from build123d import *

# Parameters (mm, degrees)
SKETCH1_W           = 20
SKETCH1_H           = 6.7
BOSS_EXTRUDE1_DEPTH = 1.5
SKETCH2_R           = 1.15
CUT_EXTRUDE1_DEPTH  = 1.5
BOSS_EXTRUDE2_DEPTH = 5
BOSS_EXTRUDE3_START = -1
BOSS_EXTRUDE3_DEPTH = 1
SKETCH5_W           = 6
SKETCH5_H           = 0.6
BOSS_EXTRUDE4_DEPTH = 4.5
SKETCH6_W           = 9
SKETCH6_H           = 1
BOSS_EXTRUDE5_DEPTH = 7.5


with BuildPart() as part:
    # Sketch1 → Boss-Extrude1 (new body)
    with BuildSketch(Plane.XY):
        Rectangle(SKETCH1_W, SKETCH1_H)
    extrude(amount=BOSS_EXTRUDE1_DEPTH)

    # Sketch2 → Cut-Extrude1 (cut)
    with BuildSketch(Plane(origin=(0, 0, 0), x_dir=(-1, 0, 0), z_dir=(0, 0, -1))):
        with Locations((-8, 0)):
            Circle(SKETCH2_R)
        with Locations((8, 0)):
            Circle(SKETCH2_R)
        with BuildLine():
            Line((-3, 1.25), (3, 1.25))
            ThreePointArc((3, 1.25), (4.25, 0), (3, -1.25))
            Line((3, -1.25), (-3, -1.25))
            ThreePointArc((-3, -1.25), (-4.25, 0), (-3, 1.25))
        make_face()
    extrude(amount=-CUT_EXTRUDE1_DEPTH, mode=Mode.SUBTRACT)

    # Sketch3 → Boss-Extrude2 (add)
    with BuildSketch(Plane.XY.offset(1.5)):
        with BuildLine():
            Line((3, 1.35), (-3, 1.35))
            ThreePointArc((-3, 1.35), (-4.35, 0), (-3, -1.35))
            Line((-3, -1.35), (3, -1.35))
            ThreePointArc((3, -1.35), (4.35, 0), (3, 1.35))
        make_face()
        with BuildLine():
            Line((3, 1.25), (-3, 1.25))
            ThreePointArc((-3, 1.25), (-4.25, 0), (-3, -1.25))
            Line((-3, -1.25), (3, -1.25))
            ThreePointArc((3, -1.25), (4.25, 0), (3, 1.25))
        make_face(mode=Mode.SUBTRACT)
    extrude(amount=BOSS_EXTRUDE2_DEPTH)

    # Sketch4 → Boss-Extrude3 (add)
    with BuildSketch(Plane.XY.offset(6.5).offset(BOSS_EXTRUDE3_START)):
        with BuildLine():
            Line((3, 1.35), (-3, 1.35))
            ThreePointArc((-3, 1.35), (-4.35, 0), (-3, -1.35))
            Line((-3, -1.35), (3, -1.35))
            ThreePointArc((3, -1.35), (4.35, 0), (3, 1.35))
        make_face()
    extrude(amount=BOSS_EXTRUDE3_DEPTH)

    # Sketch5 → Boss-Extrude4 (add)
    with BuildSketch(Plane(origin=(0, 0, 5.5), x_dir=(-1, 0, 0), z_dir=(0, 0, -1))):
        Rectangle(SKETCH5_W, SKETCH5_H)
    extrude(amount=BOSS_EXTRUDE4_DEPTH)

    # Sketch6 → Boss-Extrude5 (add)
    with BuildSketch(Plane.XY.offset(6.5)):
        Rectangle(SKETCH6_W, SKETCH6_H)
    extrude(amount=BOSS_EXTRUDE5_DEPTH)


solid = part.part
CAD build for the part. Positions are in the model's coordinates, mm. A direction names the side the tool comes from. Give positions to 0.01 mm unless a question says otherwise; leave off trailing zeros. Loops run counter-clockwise (first coordinate to the right, second up) from the corner with the lowest first, then second, coordinate; pieces in that order, holes last. Notation, with made-up numbers: M 71,-11 L 104,-11 A18 ccw 104,-4 Z; hole C 75,83 d5. An arc over 180 degrees is marked long. Answer in a Markdown table with one row per item. Add a question column.
Item 1: Drop flat-ended pins along their axis: P1, Ø0.7, axis at y = 0, z = 2, coming from the +X side; P2, Ø1, axis at x = -0.5, z = 10, coming from the +Y side; P3, Ø0.8, axis at y = 0, z = 9, coming from the +X side; P4, Ø5, axis at x = -1, z = 2.5, coming from the -Y side. Give the stop position or say it passes through.
Item 2: Band-saw the part on B-B on x = 8. Give the cut face in (y, z), then the cut area to 3 significant figures.
Item 3: Band-saw the part on A-A on z = 4.75. Give the cut face in (x, y), then the cut area to 3 significant figures.
Item 4: Mould opens along Y. For faces 6 (the face through (0, 1, 6.5)), 7 (the face through (0, -0.5, 10)), 8 (the face through (0, 0.3, 3)) say: +Y half, -Y half, draft (parallel to the pull), parting line (faces both ways), or undercut.
Item 5: Tool access for faces 1 (the face through (-4.5, 0, 10)), 2 (the face through (4.5, 0, 10)), 3 (the face through (-10, 0, 1)), 4 (the face through (0, -0.3, 3)), 5 (the face through (0, -1, 6.5)): list every direction of +Z, -Z, +X, -X, +Y, -Y with a clear straight run to the whole face (end or side of a thin tool).
Item 6: Band-saw the part on C-C on y = 0. Give the cut face in (x, z), then the cut area to 3 significant figures.
Item 7: Probe probe 1 along Y at (x, z) = (-8, 0.75); probe 2 along Y at (x, z) = (-2.5, 9); probe 3 along Z at (x, y) = (-3.25, -0.25). List the from-to ranges inside material, lowest first.
Item 8: Band-saw the part on D-D on x = 2. Give the cut face in (y, z).
Reply:
| question | item | result |
|---|---|---|
| 1 | P1 | stops at x = 4.35 |
| 1 | P2 | stops at y = 0.5 |
| 1 | P3 | stops at x = 4.5 |
| 1 | P4 | stops at y = -3.35 |
| 2 | outline | M -3.35,0 L -1.15,0 L -1.15,1.5 L -3.35,1.5 Z; M 1.15,0 L 3.35,0 L 3.35,1.5 L 1.15,1.5 Z |
| 2 | area | 6.60 mm^2 |
| 3 | outline | M -3,-1.35 L 3,-1.35 A1.35 ccw 3,1.35 L -3,1.35 A1.35 ccw Z; M -3,-0.3 L 3,-0.3 L 3,0.3 L -3,0.3 Z; hole M -3,-1.25 L 3,-1.25 A1.25 ccw 3,1.25 L -3,1.25 A1.25 ccw Z |
| 3 | area | 5.62 mm^2 |
| 4 | face 6 | draft |
| 4 | face 7 | -Y half |
| 4 | face 8 | undercut |
| 5 | face 1 | +Z, -X, +Y, -Y |
| 5 | face 2 | +Z, +X, +Y, -Y |
| 5 | face 3 | +Z, -Z, -X, +Y, -Y |
| 5 | face 4 | -Z |
| 5 | face 5 | +Z, +X, -X, -Y |
| 6 | outline | M -10,0 L -9.15,0 L -9.15,1.5 L -10,1.5 Z; M -6.85,0 L -4.25,0 L -4.25,5.5 L -3,5.5 L -3,1 L 3,1 L 3,5.5 L 4.25,5.5 L 4.25,0 L 6.85,0 L 6.85,1.5 L 4.35,1.5 L 4.35,6.5 L 4.5,6.5 L 4.5,14 L -4.5,14 L -4.5,6.5 L -4.35,6.5 L -4.35,1.5 L -6.85,1.5 Z; M 9.15,0 L 10,0 L 10,1.5 L 9.15,1.5 Z |
| 6 | area | 114 mm^2 |
| 7 | probe 1 | y = -3.35 to -1.15, 1.15 to 3.35 |
| 7 | probe 2 | y = -0.5 to 0.5 |
| 7 | probe 3 | z = 5.5 to 14 |
| 8 | outline | M -3.35,0 L -1.25,0 L -1.25,5.5 L -0.3,5.5 L -0.3,1 L 0.3,1 L 0.3,5.5 L 1.25,5.5 L 1.25,0 L 3.35,0 L 3.35,1.5 L 1.35,1.5 L 1.35,6.5 L 0.5,6.5 L 0.5,14 L -0.5,14 L -0.5,6.5 L -1.35,6.5 L -1.35,1.5 L -3.35,1.5 Z |
